```python
from build123d import *

# Parameters (mm, degrees)
SKETCH1_W           = 44
SKETCH1_H           = 27.7
BOSS_EXTRUDE1_DEPTH = 10
SKETCH2_W           = 13.15
SKETCH2_H           = 27.7
BOSS_EXTRUDE2_DEPTH = 25
SKETCH3_R           = 2.5
CUT_EXTRUDE1_DEPTH  = 10
SKETCH4_W           = 0.76
SKETCH4_H           = 27.7
CUT_EXTRUDE2_DEPTH  = 2.2


with BuildPart() as part:
    # Sketch1 → Boss-Extrude1 (new body)
    with BuildSketch(Plane.XY):
        Rectangle(SKETCH1_W, SKETCH1_H)
    extrude(amount=BOSS_EXTRUDE1_DEPTH)

    # Sketch2 → Boss-Extrude2 (add)
    with BuildSketch(Plane(origin=(0, 0, 0), x_dir=(-1, 0, 0), z_dir=(0, 0, -1))):
        with Locations((-15.425, 0)):
            Rectangle(SKETCH2_W, SKETCH2_H)
        with Locations((15.425, 0)):
            Rectangle(SKETCH2_W, SKETCH2_H)
    extrude(amount=BOSS_EXTRUDE2_DEPTH)

    # Sketch3 → Cut-Extrude1 (cut)
    with BuildSketch(Plane.XY.offset(10)):
        Circle(SKETCH3_R)
    extrude(amount=-CUT_EXTRUDE1_DEPTH, mode=Mode.SUBTRACT)

    # Sketch4 → Cut-Extrude2 (cut)
    with BuildSketch(Plane(origin=(0, 0, 0), x_dir=(-1, 0, 0), z_dir=(0, 0, -1))):
        with Locations((-8.47, 0)):
            Rectangle(SKETCH4_W, SKETCH4_H)
        with Locations((8.47, 0)):
            Rectangle(SKETCH4_W, SKETCH4_H)
    extrude(amount=-CUT_EXTRUDE2_DEPTH, mode=Mode.SUBTRACT)


solid = part.part
```
The model under review builds one solid part; all positions refer to its coordinate system, in mm. A direction names the side the tool comes from. Coordinates: 2 decimals unless noted, no trailing zeros. Write each loop counter-clockwise with the first axis right and the second up, starting at its lowest first coordinate (ties: lowest second). Pieces come first, ordered by that corner, then holes. Notation, with made-up numbers: (51, 47.25) -> (73, 47.25) arc R24 cw to (73, 73.25) -> close; hole circle Ø8 at (89, 52.25). An arc over 180 degrees is marked (long way). One line per item, written item: value. Start each with the question number.
Q1. To check wall thickness, follow probe 1 along Y at (x, z) = (0, 6.25); probe 2 along X at (y, z) = (8.25, -22); probe 3 along Z at (x, y) = (-3.5, 8). State the ranges of each line that lie inside material, in increasing order.
Q2. Add section A-A, the plane z = -10.5. Give the boundary of the cut face in (x, y).
Q3. Add section D-D, the plane z = 7. Give the boundary of the cut face in (x, y).
Q4. Clearance check with flat-ended pins moving along their axes: P1, Ø1, axis at x = 4.5, y = -8.5, coming from the -Z side; P2, Ø0.6, axis at x = -8.5, y = -5, coming from the -Z side. State where each tip first meets the part, or that it passes through.
Q5. Add section C-C, the plane x = 0. Give the boundary of the cut face in (y, z).
Q6. For faces 1 (the face through (-8.09, 0, 1)), 2 (the face through (16, 0, -25)), list the 3-axis set-ups (+Z, -Z, +X, -X, +Y, -Y) from which the entire face can be reached by the end or side of a thin tool; tool diameter is ignored.
Q7. Add section B-B, the plane y = 0. Give the boundary of the cut face in (x, z).
Q8. The part is to be moulded in two halves that separate along Y. For faces 3 (the face through (-0.54, -2.44, 5.07)), 4 (the face through (0, 13.85, 1)), 5 (the face through (-22, 0, -8)), say which applies: +Y half, -Y half, draft (parallel to the pull), parting line (faces both ways), or undercut.
Response:
1. probe 1: -13.85 to -2.5, 2.5 to 13.85
1. probe 2: -22 to -8.85, 8.85 to 22
1. probe 3: 0 to 10
2. outline: (-22, -13.85) -> (-8.85, -13.85) -> (-8.85, 13.85) -> (-22, 13.85) -> close; (8.85, -13.85) -> (22, -13.85) -> (22, 13.85) -> (8.85, 13.85) -> close
3. outline: (-22, -13.85) -> (22, -13.85) -> (22, 13.85) -> (-22, 13.85) -> close; hole circle Ø5 at (0, 0)
4. P1: z = 0
4. P2: z = 2.2
5. outline: (-13.85, 0) -> (-2.5, 0) -> (-2.5, 10) -> (-13.85, 10) -> close; (2.5, 0) -> (13.85, 0) -> (13.85, 10) -> (2.5, 10) -> close
6. face 1: -Z, +Y, -Y
6. face 2: -Z, +X, -X, +Y, -Y
7. outline: (-22, -25) -> (-8.85, -25) -> (-8.85, 2.2) -> (-8.09, 2.2) -> (-8.09, 0) -> (-2.5, 0) -> (-2.5, 10) -> (-22, 10) -> close; (2.5, 0) -> (8.09, 0) -> (8.09, 2.2) -> (8.85, 2.2) -> (8.85, -25) -> (22, -25) -> (22, 10) -> (2.5, 10) -> close
8. face 3: undercut
8. face 4: +Y half
8. face 5: draft
